Input: dimensioned drawing with shaded views. Units: mm. Origin: part minimum x, y, z. A direction names the side the tool comes from. Round coordinates to 2 decimals unless told otherwise and drop trailing zeros. Loops run counter-clockwise (first coordinate to the right, second up) from the corner with the lowest first, then second, coordinate; pieces in that order, holes last. Notation, with made-up numbers: (-0.5, 22.5) - (7.5, 22.5) arc R13 ccw to (7.5, 39.5) - close; hole circle Ø1 at (47, 37). An arc over 180 degrees is marked (long way). Use CSV: the item, a comma, the result in double quotes. Start each with the question number.
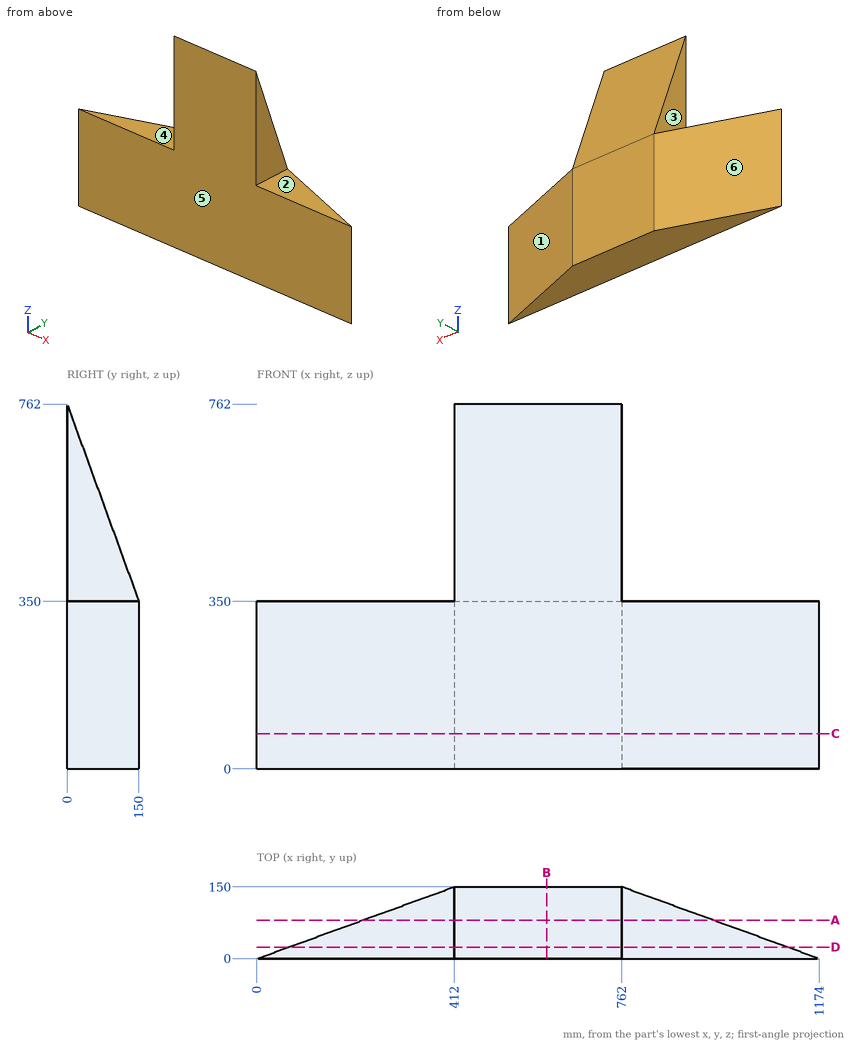
1. Mould query, pull axis Y, two halves, no side actions, for the marked faces 4, 5 and 6. Classes: +Y half, -Y half, draft (parallel to the pull), parting line (faces both ways), or undercut.
2. Section query A-A on y = 80.5. Return the cut outline in (x, z), and give its area (3 significant figures).
3. Section query D-D on y = 24. Return the cut outline in (x, z).
4. Section query C-C on z = 73.5. Return the cut outline in (x, y).
5. Line query: line 1 along X through (y, z) = (28, 594); line 2 along Z through (x, y) = (1019, 23); line 3 along Y through (x, z) = (803, 115.5). Output: solid intervals per line, ascending.
6. Reachability of the marked faces 1, 2 and 3 from +Z, -Z, +X, -X, +Y, -Y: full face, straight path, thin tool, end or side. Return the list, or none.
7. Section query B-B on x = 605. Return the cut outline in (y, z).
8. Contact query for a flat-ended pin moving along its axis: P1, Ø1.5, axis at x = 157.5, y = 16.5, coming from the +Z side. Output: stop coordinate, or through.
Values:
1,face 4,"draft"
1,face 5,"-Y half"
1,face 6,"+Y half"
2,outline,"(221.11, 0) - (952.89, 0) - (952.89, 350) - (762, 350) - (762, 540.89) - (412, 540.89) - (412, 350) - (221.11, 350) - close"
2,area,"323,000 mm^2"
3,outline,"(65.92, 0) - (1108.08, 0) - (1108.08, 350) - (762, 350) - (762, 696.08) - (412, 696.08) - (412, 350) - (65.92, 350) - close"
4,outline,"(0, 0) - (1174, 0) - (762, 150) - (412, 150) - close"
5,line 1,"x = 412 to 762"
5,line 2,"z = 0 to 350"
5,line 3,"y = 0 to 135.07"
6,face 1,"+Z, -Z, +X, +Y"
6,face 2,"+Z, +X, +Y, -Y"
6,face 3,"+Z, -X, +Y, -Y"
7,outline,"(0, 0) - (150, 0) - (150, 350) - (0, 762) - close"
8,P1,"stops at z = 350"
